Job drawing, mm, ordinate dimensions from the low corner. One solid piece. Coordinates: 2 decimals unless noted, no trailing zeros. Loops run counter-clockwise (first coordinate to the right, second up) from the corner with the lowest first, then second, coordinate; pieces in that order, holes last. Notation, with made-up numbers: M -40,85 L -24,85 A9 cw -24,90 Z; hole C 41,-13 d9. An arc over 180 degrees is marked long. Answer as a JSON object with one key per item and string values. Group by question number.
1. Saw through at B-B on z = 8. Write the cut outline in (x, y), then the cut area to 3 significant figures.
2. Drop flat-ended pins along their axis: pin 1 Ø5 at (x, z) = (8, 52) entering from +Y; pin 2 Ø3.5 at (x, z) = (92, 52) entering from +Y. Give the stop position or say it passes through.
3. Saw through at A-A on x = 8. Write the cut outline in (y, z), then the cut area to 3 significant figures.
4. Drill centre lines: L1, parallel to Z at x = 92, y = 1.55; L2, parallel to X at y = 2.2, z = 6; L3, parallel to X at y = 0.8, z = 57.5. Where is each one in solid material? Low to high.
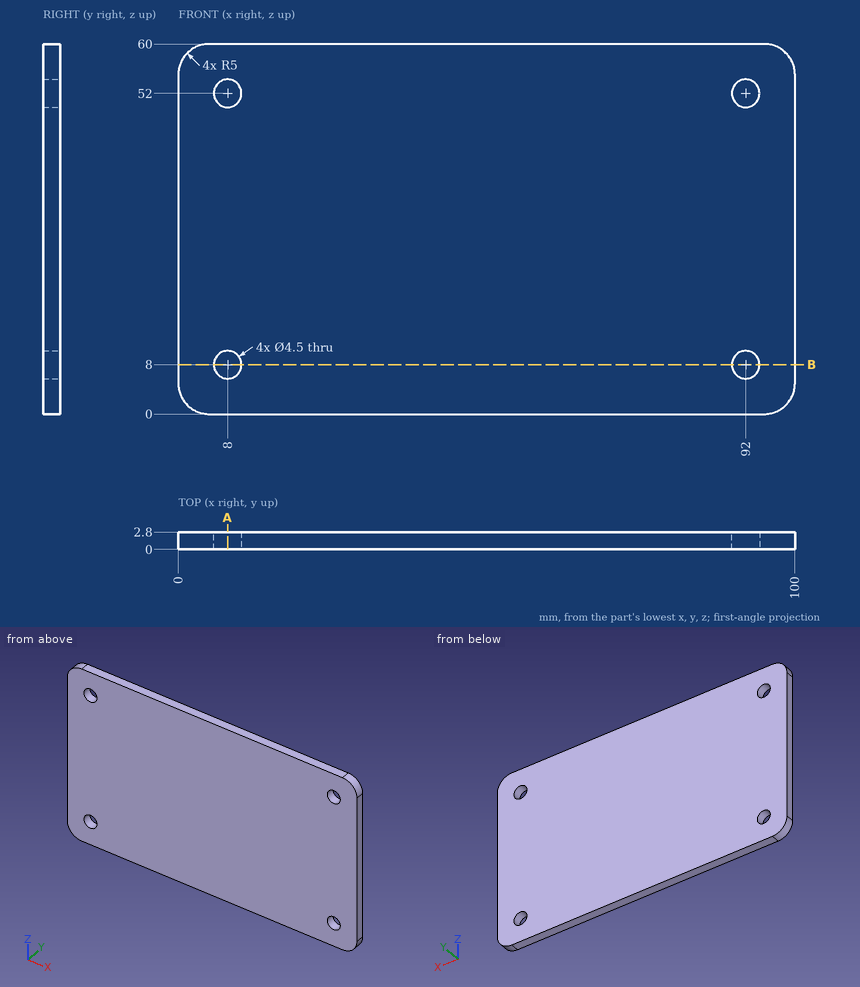
Outcome:
{
 "1": {"outline": "M 0,0 L 5.75,0 L 5.75,2.8 L 0,2.8 Z; M 10.25,0 L 89.75,0 L 89.75,2.8 L 10.25,2.8 Z; M 94.25,0 L 100,0 L 100,2.8 L 94.25,2.8 Z", "area": "255 mm²"},
 "2": {"pin 1": "stops at y = 2.8", "pin 2": "passes through"},
 "3": {"outline": "M 0,0 L 2.8,0 L 2.8,5.75 L 0,5.75 Z; M 0,10.25 L 2.8,10.25 L 2.8,49.75 L 0,49.75 Z; M 0,54.25 L 2.8,54.25 L 2.8,60 L 0,60 Z", "area": "143 mm²"},
 "4": {"L1": "z = 0 to 5.75, 10.25 to 49.75, 54.25 to 60", "L2": "x = 0 to 6.97, 9.03 to 90.97, 93.03 to 100", "L3": "x = 0.67 to 99.33"}
}
